```python
from build123d import *

# Parameters (mm, degrees)
SKETCH1_W           = 48.26
SKETCH1_H           = 17.78
BOSS_EXTRUDE1_DEPTH = 17.579999892
BOSS_EXTRUDE4_DEPTH = 46.720000032
CUT_EXTRUDE1_DEPTH  = 70.432286432
BOSS_EXTRUDE5_DEPTH = 46.72
SKETCH9_W           = 0.75
SKETCH9_H           = 25.854438162


with BuildPart() as part:
    # Sketch1 → Boss-Extrude1 (new body)
    with BuildSketch(Plane.XY):
        with Locations((24.13, 8.89)):
            Rectangle(SKETCH1_W, SKETCH1_H)
    extrude(amount=-BOSS_EXTRUDE1_DEPTH)

    # Sketch3 → Boss-Extrude4 (add)
    with BuildSketch(Plane(origin=(0, 17.78, 0), x_dir=(1, 0, 0), z_dir=(0, 1, 0))):
        Polygon((37.801769271, 9.565696577), (37.128446266, 10.181556346), (37.128446266, 0), (48.26, 0), (48.26, 13.587965792), (48.26, 17.579999892), (45.132109917, 17.579999892), align=None)
    extrude(amount=BOSS_EXTRUDE4_DEPTH)

    # Sketch4 → Cut-Extrude1 (cut, through all)
    with BuildSketch(Plane(origin=(0, 17.78, 0), x_dir=(1, 0, 0), z_dir=(0, 1, 0))):
        with BuildLine():
            Line((30.48, 6.789), (22.86, 6.789))
            ThreePointArc((22.86, 6.789), (20.86, 8.789), (22.86, 10.789))
            Line((22.86, 10.789), (30.48, 10.789))
            ThreePointArc((30.48, 10.789), (32.48, 8.789), (30.48, 6.789))
        make_face()
        with BuildLine():
            Line((13.78, 6.789), (6.16, 6.789))
            ThreePointArc((6.16, 6.789), (4.16, 8.789), (6.16, 10.789))
            Line((6.16, 10.789), (13.78, 10.789))
            ThreePointArc((13.78, 10.789), (15.78, 8.789), (13.78, 6.789))
        make_face()
    extrude(amount=-CUT_EXTRUDE1_DEPTH, mode=Mode.SUBTRACT)

    # Sketch3<7> → Boss-Extrude5 (add, through all)
    with BuildSketch(Plane(origin=(0, 17.78, 0), x_dir=(1, 0, 0), z_dir=(0, 1, 0))):
        Polygon((54.944699529, 28.308160187), (54.271376524, 28.924019957), (37.128446266, 10.181556346), (37.801769271, 9.565696577), align=None)
    extrude(amount=BOSS_EXTRUDE5_DEPTH)

    # Sketch9 → Ø1.5mm Dowel Hole1 (revolve, cut)
    with BuildSketch(Plane(origin=(41.16709667, 56.699990232, -6.487575467), x_dir=(0.7378922681206892, 0, 0.6749185140798146), z_dir=(0, 1, 0))):
        with Locations((0.375, 12.927219081)):
            Rectangle(SKETCH9_W, SKETCH9_H)
    revolve(axis=Axis((36.881364106, 56.699990232, -1.801959564), (0.6749185140798145, 0, -0.7378922681206892)), mode=Mode.SUBTRACT)


solid = part.part
```
Input: part model. Units: mm. Frame: model coordinates. A direction names the side the tool comes from. Give positions to 0.01 mm unless a question says otherwise; leave off trailing zeros. Order: outer loops, then holes, each group sorted by start corner. A loop starts at its lowest first (then second) coordinate and runs counter-clockwise, first axis right, second up. Notation, with made-up numbers: (-31, 45) - (12, 45) arc R18 cw to (12, 61) - close; hole circle Ø10 at (19, 16.5). An arc over 180 degrees is marked (long way). One line per item, written item: value.
1. Cut plane D-D, the plane y = 23.5. Output: boundary loops of the cut face in (x, z), and give its area (3 significant figures).
Determined:
outline: (37.13, -10.18) - (54.27, -28.92) - (54.94, -28.31) - (45.13, -17.58) - (48.26, -17.58) - (48.26, 0) - (37.13, 0) - close
area: 184 mm2
2. Reachability of faces 4 (the face through (37.128, 41, -5)), 5 (the face through (10, 9, -10.789)), 6 (the face through (50, 40.8, -22.9)), 7 (the face through (45.82, 40.813, -19.684)) from +Z, -Z, +X, -X, +Y, -Y: full face, straight path, thin tool, end or side. Return the list, or none.
Determined:
face 4: +Z, -Z, -X, +Y
face 5: +Y, -Y
face 6: +X, +Y, -Y
face 7: -Z, -X, +Y
3. Line query: probe 1 along X at (y, z) = (3.5, -1.5); probe 2 along Y at (x, z) = (30.5, -6.75); probe 3 along Z at (x, y) = (47, 14). Output: solid intervals per line, ascending.
Determined:
probe 1: 0 to 48.26
probe 2: 0 to 17.78
probe 3: -17.58 to 0
4. Pin query (flat end, axial travel): pin 1 Ø5.5 at (x, z) = (26, -7) entering from +Y; pin 2 Ø12 at (y, z) = (40.5, -3) entering from -X; pin 3 Ø1 at (x, z) = (45, -18) entering from -Y; pin 4 Ø1.5 at (y, z) = (29, -17) entering from -X. Return the tip coordinate at first contact, or that it passes through.
Determined:
pin 1: y = 17.78
pin 2: x = 37.13
pin 3: y = 0
pin 4: x = 42.68
5. Cut plane B-B, the plane y = 13.5. Output: boundary loops of the cut face in (x, z).
Determined:
outline: (0, -17.58) - (48.26, -17.58) - (48.26, 0) - (0, 0) - close; hole (6.16, -10.79) - (13.78, -10.79) arc R2 ccw to (13.78, -6.79) - (6.16, -6.79) arc R2 ccw to start; hole (22.86, -10.79) - (30.48, -10.79) arc R2 ccw to (30.48, -6.79) - (22.86, -6.79) arc R2 ccw to start
6. Draft query along Y for faces 1 (the face through (44.517, 56.667, -11.261)), 2 (the face through (49.8, 17.78, -23.3)), 3 (the face through (48.26, 32, -9)). Return one class per face: released by +Y, released by -Y, zero draft, split by the parting line, or undercut.
Determined:
face 1: undercut
face 2: released by -Y
face 3: zero draft
7. Cut plane A-A, the plane x = 9. Output: boundary loops of the cut face in (y, z), and give its area (3 significant figures).
Determined:
outline: (0, -17.58) - (17.78, -17.58) - (17.78, -10.79) - (0, -10.79) - close; (0, -6.79) - (17.78, -6.79) - (17.78, 0) - (0, 0) - close
area: 241 mm2
8. Cut plane C-C, the plane z = -3.75. Output: boundary loops of the cut face in (x, y).
Determined:
outline: (0, 0) - (48.26, 0) - (48.26, 64.5) - (37.13, 64.5) - (37.13, 17.78) - (0, 17.78) - close
